Geometry check sheet. Reference: the model listing, model coordinates, mm. Round coordinates to 2 decimals unless told otherwise and drop trailing zeros. Write each loop counter-clockwise with the first axis right and the second up, starting at its lowest first coordinate (ties: lowest second). Pieces come first, ordered by that corner, then holes.
Item 1: Cross-section at A-A (x = 50.9). Enter the section's corners in (y, z).
Item 2: Cross-section at B-B (y = 0). Enter the section's corners in (x, z), then the cut area to 3 significant figures.
Item 3: Cross-section at C-C (z = -1.5). Enter the section's corners in (x, y).
Item 4: Cross-section at D-D (x = -53). Enter the section's corners in (y, z), then the cut area to 3 significant figures.
Item 5: Scan lines: probe 1 along X at (y, z) = (0, 2.75); probe 2 along Y at (x, z) = (-50.9, -1.25); probe 3 along X at (y, z) = (-2.5, -3.75). Record each from-to range of solid material in increasing order.
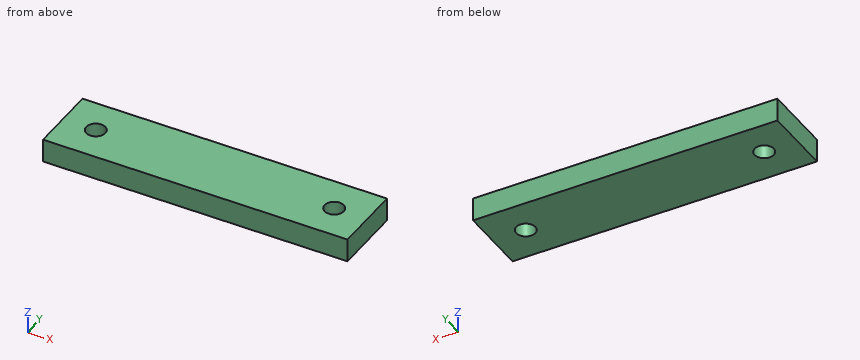
Autodesk Inventor part; units mm, degrees
ref_plane "YZ Plane" through (0, 0, 0) normal (1, 0, 0) x (0, 1, 0)
ref_plane "XZ Plane" through (0, 0, 0) normal (0, 1, 0) x (-1, 0, 0)
ref_plane "XY Plane" through (0, 0, 0) normal (0, 0, 1) x (1, 0, 0)
sketch "Sketch1" plane through (0, 0, 0) normal (0, 0, 1) x (1, 0, 0)
  line L0 (0, 21) -> (0, -21) construction
  line L1 (-91, 0) -> (91, 0) construction
  line L2 (65, -15) -> (-65, -15)
  line L3 (-65, -15) -> (-65, 15)
  line L4 (-65, 15) -> (65, 15)
  line L5 (65, 15) -> (65, -15)
  line L6 (65, -15) -> (-65, 15) construction
  line L7 (-65, -15) -> (65, 15) construction
  point P0 (0, 0)
  dimension "d4" = 130
  dimension "d5" = 30
extrude "Extrusion3" add sketch "Sketch1" along normal mid plane 10
sketch "Sketch2" plane through (0, 0, -5) normal (0, 0, -1) x (-1, 0, 0)
  point P0 (0, 0)
  point P1 (-50.9, 0)
  point P2 (50.9, 0)
  dimension "d8" = 101.8
  dimension "d9" = 50.9
hole "Hole1" at (50.9, 0, -5) at (-50.9, 0, -5) direction (0, 0, 1) diameter 8.2 end through all
properties part number "17-0028-0035" material "Copper"
Resolved:
1. outline: (-15, -5) - (-4.1, -5) - (-4.1, 5) - (-15, 5) - close; (4.1, -5) - (15, -5) - (15, 5) - (4.1, 5) - close
2. outline: (-65, -5) - (-55, -5) - (-55, 5) - (-65, 5) - close; (-46.8, -5) - (46.8, -5) - (46.8, 5) - (-46.8, 5) - close; (55, -5) - (65, -5) - (65, 5) - (55, 5) - close
2. area: 1,140 mm2
3. outline: (-65, -15) - (65, -15) - (65, 15) - (-65, 15) - close; hole circle Ø8.2 at (-50.9, 0); hole circle Ø8.2 at (50.9, 0)
4. outline: (-15, -5) - (-3.52, -5) - (-3.52, 5) - (-15, 5) - close; (3.52, -5) - (15, -5) - (15, 5) - (3.52, 5) - close
4. area: 230 mm2
5. probe 1: x = -65 to -55, -46.8 to 46.8, 55 to 65
5. probe 2: y = -15 to -4.1, 4.1 to 15
5. probe 3: x = -65 to -54.15, -47.65 to 47.65, 54.15 to 65
